from build123d import *

# Parameters (mm, degrees)
SKETCH1_W           = 14
SKETCH1_H           = 30
BOSS_EXTRUDE1_DEPTH = 30
SKETCH2_W           = 14
SKETCH2_H           = 2.25
BOSS_EXTRUDE2_DEPTH = 5
SKETCH3_R           = 1.5
CUT_EXTRUDE1_DEPTH  = 31.725600076
SKETCH4_R           = 3
BOSS_EXTRUDE3_DEPTH = 5
CHAMFER1_SIZE       = 5
CHAMFER1_SIZE2      = 15
FILLET1_R           = 2
FILLET2_R           = 0.5


with BuildPart() as part:
    # Sketch1 → Boss-Extrude1 (new body)
    with BuildSketch(Plane(origin=(0, 0, 0), x_dir=(1, 0, 0), z_dir=(0, 1, 0))):
        Rectangle(SKETCH1_W, SKETCH1_H)
    extrude(amount=BOSS_EXTRUDE1_DEPTH)

    # Sketch2 → Boss-Extrude2 (add)
    with BuildSketch(Plane.XY.offset(15)):
        with Locations((0, 21.125)):
            Rectangle(SKETCH2_W, SKETCH2_H)
    boss_extrude2 = extrude(amount=BOSS_EXTRUDE2_DEPTH)

    # Sketch3 → Cut-Extrude1 (cut, through all)
    with BuildSketch(Plane(origin=(0, 22.25, 0), x_dir=(1, 0, 0), z_dir=(0, 1, 0))):
        with Locations(Location((0, -17.5, 0), (0, 0, 270))):
            Circle(SKETCH3_R)
    cut_extrude1 = extrude(amount=-CUT_EXTRUDE1_DEPTH, mode=Mode.SUBTRACT)

    # Mirror1: Boss-Extrude2, Cut-Extrude1 across plane
    add(boss_extrude2.mirror(Plane.XY))
    add(cut_extrude1.mirror(Plane.XY), mode=Mode.SUBTRACT)

    # Sketch4 → Boss-Extrude3 (add)
    with BuildSketch(Plane(origin=(0, 30, 0), x_dir=(1, 0, 0), z_dir=(0, 1, 0))):
        with Locations(Location((0, -9, 0), (0, 0, 90))):
            Circle(SKETCH4_R)
    extrude(amount=BOSS_EXTRUDE3_DEPTH)

    # Chamfer1
    chamfer1_edges = [part.edges().sort_by_distance(p)[0] for p in [
        (0, 30, -15),
    ]]
    chamfer1_side = [part.faces().sort_by_distance(p)[0] for p in [
        (0, 26.125, -15),
    ]]
    chamfer(chamfer1_edges, length=CHAMFER1_SIZE, length2=CHAMFER1_SIZE2, reference=chamfer1_side[0])

    # Fillet1
    fillet1_edges = [part.edges().sort_by_distance(p)[0] for p in [
        (-7, 21.125, 20),
        (7, 21.125, 20),
        (-7, 21.125, -20),
        (7, 21.125, -20),
    ]]
    fillet(fillet1_edges, radius=FILLET1_R)

    # Fillet2
    fillet2_edges = [part.edges().sort_by_distance(p)[0] for p in [
        (0, 30, 15),
        (7, 10, 15),
        (-7, 10, 15),
        (-7, 10, -15),
        (7, 10, -15),
        (7, 30, 7.5),
        (0, 0, 15),
        (-7, 0, 0),
        (0, 0, -15),
        (7, 0, 0),
        (-7, 30, 7.5),
        (0, 30, 0),
        (-7, 23.625, -15),
        (-7, 27.5, -7.5),
        (7, 23.625, -15),
        (0, 25, -15),
        (7, 27.5, -7.5),
        (7, 26.125, 15),
        (-7, 26.125, 15),
    ]]
    fillet(fillet2_edges, radius=FILLET2_R)


solid = part.part
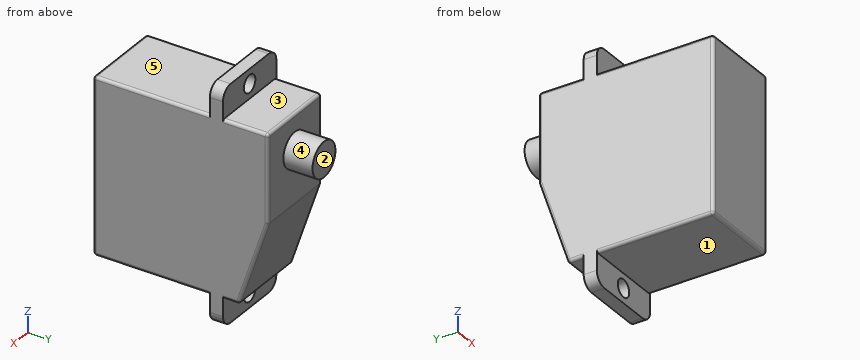
Read the model definition and answer for the solid it produces. Units are mm, in the model's axes. Face numbers are marked on the shaded views. A direction names the side the tool comes from. Coordinates: 2 decimals unless noted, no trailing zeros. Order: outer loops, then holes, each group sorted by start corner. A loop starts at its lowest first (then second) coordinate and runs counter-clockwise, first axis right, second up. Notation, with made-up numbers: M 87,89 L 118,89 A33 cw 118,122 Z; hole C 46.25,58 d4. An arc over 180 degrees is marked long. Put each result on its own line as item: value. Start each with the question number.
Item 1: Section C-C, the plane y = 3 is taken. Determine the outline of the cut face in (x, z).
Item 2: Section D-D, the plane z = 9 is taken. Determine the outline of the cut face in (x, y).
Item 3: Given pin 1 Ø4.5 at (x, z) = (0, -16) entering from +Y; pin 2 Ø1.9 at (x, y) = (-2.5, 24) entering from -Z; pin 3 Ø2 at (x, y) = (4, 6.5) entering from +Z, each flat-ended and moving along its own axis, determine where each tip first touches the part or whether it passes through.
Item 4: Section B-B, the plane x = 4.5 is taken. Determine the outline of the cut face in (y, z).
Item 5: For the marked faces 1, 2, 3, 4 and 5, determine the directions among +Z, -Z, +X, -X, +Y, -Y from which every point of the face is accessible in a straight line to the end or side of a thin tool.
Item 6: Section A-A, the plane z = 17.5 is taken. Determine the outline of the cut face in (x, y).
Item 7: Consider probe 1 along X at (y, z) = (21.2, -17.5); probe 2 along Z at (x, y) = (2.25, 5); probe 3 along Y at (x, z) = (-3.25, 14). Determine where each line is inside the solid, lowest interval first. Write a range as [from, to].
Computed:
1. outline: M -7,-14.5 A0.5 ccw -6.5,-15 L 6.5,-15 A0.5 ccw 7,-14.5 L 7,14.5 A0.5 ccw 6.5,15 L -6.5,15 A0.5 ccw -7,14.5 Z
2. outline: M -7,0.5 A0.5 ccw -6.5,0 L 6.5,0 A0.5 ccw 7,0.5 L 7,29.5 A0.5 ccw 6.5,30 L 3,30 L 3,35 L -3,35 L -3,30 L -6.5,30 A0.5 ccw -7,29.5 Z
3. pin 1: stops at y = 25.42
3. pin 2: stops at z = -15
3. pin 3: stops at z = 15
4. outline: M 0,-14.5 A0.5 ccw 0.5,-15 L 20,-15 L 20,-20 L 22.25,-20 L 22.25,-15 L 24.64,-15 A0.5 ccw 25.11,-14.66 L 29.97,-0.08 A0.5 ccw 30,0.08 L 30,14.5 A0.5 ccw 29.5,15 L 22.25,15 L 22.25,20 L 20,20 L 20,15 L 0.5,15 A0.5 ccw 0,14.5 Z
5. face 1: -Z, +X, -X, -Y
5. face 2: +Z, -Z, +X, -X, +Y
5. face 3: +Z, +X, -X, +Y
5. face 4: +Y
5. face 5: +Z, +X, -X, -Y
6. outline: M -7,20 L -1.5,20 L -1.5,22.25 L -7,22.25 Z; M 1.5,20 L 7,20 L 7,22.25 L 1.5,22.25 Z
7. probe 1: x = [-7, -1.5], [1.5, 7]
7. probe 2: z = [-15, 15]
7. probe 3: y = [0, 30]
